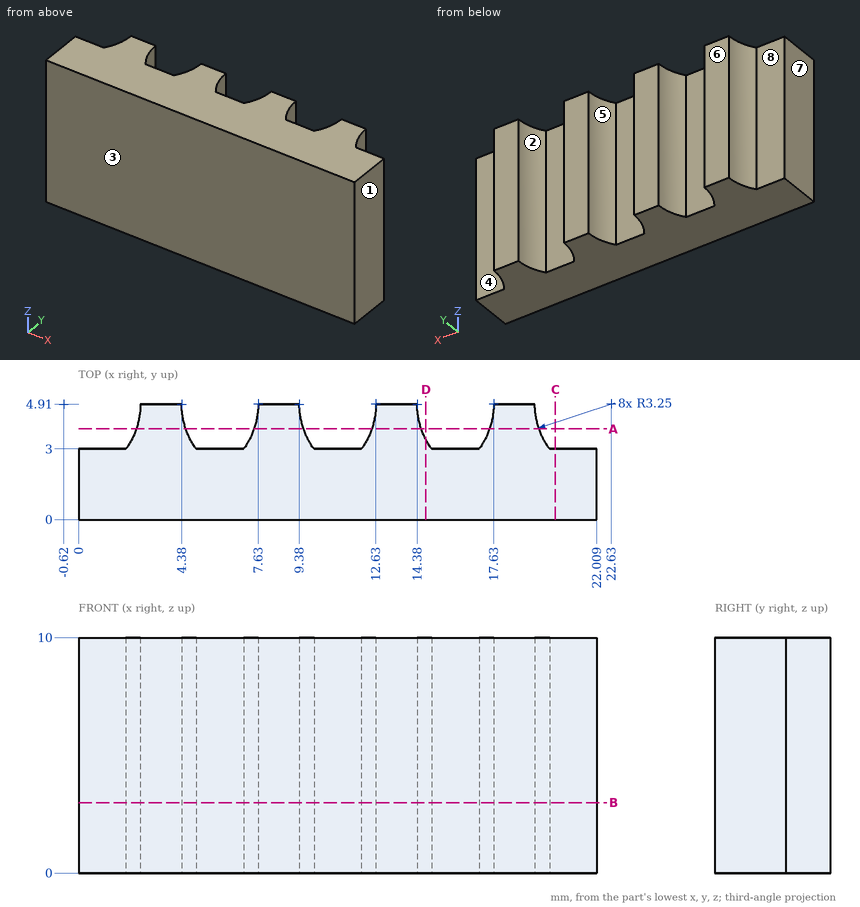
The figure shows three views and two pictorial views of one solid part (mm, origin at its lowest corner). Answer the questions. A direction names the side the tool comes from. Give positions to 0.01 mm unless a question says otherwise; leave off trailing zeros. Order: outer loops, then holes, each group sorted by start corner. A loop starts at its lowest first (then second) coordinate and runs counter-clockwise, first axis right, second up. Notation, with made-up numbers: (59.5, -29) -> (63.5, -29) arc R29 ccw to (63.5, 3) -> close; hole circle Ø8 at (-0.75, 11). An arc over 180 degrees is marked (long way). Answer as a JSON object with one key per item and string values. Group by question number.
Item 1: The part is cut by section B-B on z = 3. Write down the section's boundary in (x, y).
Item 2: Determine the mould class of the marked faces 1, 2 and 3 for opening direction X: pulls with the +X half, pulls with the -X half, needs draft (parallel to the pull), parting line crosses it, or undercut.
Item 3: The part is cut by section D-D on x = 14.75. Write down the section's boundary in (y, z), and give its area (3 significant figures).
Item 4: Flat-ended cylindrical pins translate along their axes: pin 1 (1.5 mm diameter, centred on x = 14, z = 8.5, fed in from -Y); pin 2 (0.6 mm diameter, centred on x = 0.5, z = 4.5, fed in from +Y). Find the tip coordinate at first contact, or state that the pin passes through.
Item 5: Consider L1, parallel to X at y = 4.6, z = 1.25 (1 decimal); L2, parallel to Y at x = 16.5, z = 5.5; L3, parallel to X at y = 3.35, z = 4. Determine where each line is inside the solid, lowest interval first. Write a range as from..to.
Item 6: The part is cut by section C-C on x = 20.25. Write down the section's boundary in (y, z), and give its area (3 significant figures).
Item 7: The part is cut by section A-A on y = 3.85. Write down the section's boundary in (x, z).
Item 8: A tool of negligible diameter and unlimited length cuts with its end or side. For the marked faces 4, 5, 6, 7 and 8, from which of +Z, -Z, +X, -X, +Y, -Y can it reach the whole face along a straight path? Write none if from no direction.
Result set:
{
 "1": {"outline": "(0, 0) -> (22.01, 0) -> (22.01, 3) -> (20, 3) arc R3.25 cw to (19.38, 4.91) -> (17.63, 4.91) arc R3.25 cw to (17.01, 3) -> (15, 3) arc R3.25 cw to (14.38, 4.91) -> (12.63, 4.91) arc R3.25 cw to (12.01, 3) -> (10, 3) arc R3.25 cw to (9.38, 4.91) -> (7.63, 4.91) arc R3.25 cw to (7.01, 3) -> (5, 3) arc R3.25 cw to (4.38, 4.91) -> (2.63, 4.91) arc R3.25 cw to (2.01, 3) -> (0, 3) -> close"},
 "2": {"face 1": "pulls with the +X half", "face 2": "undercut", "face 3": "needs draft"},
 "3": {"outline": "(0, 0) -> (3.4, 0) -> (3.4, 10) -> (0, 10) -> close", "area": "34.0 mm²"},
 "4": {"pin 1": "y = 0", "pin 2": "y = 3"},
 "5": {"L1": "2.6..4.4, 7.6..9.4, 12.6..14.4, 17.6..19.4", "L2": "0..3", "L3": "2.23..4.78, 7.23..9.78, 12.23..14.78, 17.23..19.78"},
 "6": {"outline": "(0, 0) -> (3, 0) -> (3, 10) -> (0, 10) -> close", "area": "30.0 mm²"},
 "7": {"outline": "(2.45, 0) -> (4.56, 0) -> (4.56, 10) -> (2.45, 10) -> close; (7.45, 0) -> (9.56, 0) -> (9.56, 10) -> (7.45, 10) -> close; (12.45, 0) -> (14.56, 0) -> (14.56, 10) -> (12.45, 10) -> close; (17.45, 0) -> (19.56, 0) -> (19.56, 10) -> (17.45, 10) -> close"},
 "8": {"face 4": "+Z, -Z, +X, +Y", "face 5": "+Z, -Z, +Y", "face 6": "+Z, -Z, +X, -X, +Y", "face 7": "+Z, -Z, -X, +Y, -Y", "face 8": "+Z, -Z, -X, +Y"}
}
